from build123d import *

# Parameters (mm, degrees)
F0_W     = 50.8
F0_H     = 38.1
F1_DEPTH = 12.7
F3_DEPTH = 12.7
F5_DEPTH = 12.7
F6_R     = 6.3499999233
F7_DEPTH = 25.401
F8_R     = 6.35
F9_DEPTH = 12.701
F10_R    = 12.7


with BuildPart() as f1:
    # F0 (on Top) → F1 (new body)
    with BuildSketch(Plane.XY):
        Rectangle(F0_W, F0_H)
    extrude(amount=F1_DEPTH)

    # F2 (on face) → F3 (join)
    with BuildSketch(Plane(origin=(0, 19.05, 0), x_dir=(-1, 0, 0), z_dir=(0, 1, 0))):
        with BuildLine():
            ThreePointArc((-12.7, 26.0490588844), (-17.3287683055, 17.7369875968), (-25.4, 12.7))
            Line((-25.4, 12.7), (-12.7, 12.7))
            Line((-12.7, 12.7), (12.7, 12.7))
            Line((12.7, 12.7), (25.4, 12.7))
            ThreePointArc((25.4, 12.7), (17.3287683055, 17.7369875968), (12.7, 26.0490588844))
            Line((12.7, 26.0490588844), (12.7, 69.85))
            ThreePointArc((12.7, 69.85), (0, 57.15), (-12.7, 69.85))
            Line((-12.7, 69.85), (-12.7, 26.0490588844))
        make_face()
        with BuildLine():
            ThreePointArc((12.7, 69.85), (0, 82.55), (-12.7, 69.85))
            ThreePointArc((-12.7, 69.85), (0, 57.15), (12.7, 69.85))
        make_face()
    extrude(amount=-F3_DEPTH)

    # F4 (on face) → F5 (join)
    with BuildSketch(Plane.XZ.offset(-6.35)):
        with BuildLine():
            ThreePointArc((-12.7, 69.85), (0, 57.15), (12.7, 69.85))
            ThreePointArc((12.7, 69.85), (0, 82.55), (-12.7, 69.85))
        make_face()
    extrude(amount=F5_DEPTH)

    # F6 (on face) → F7 (cut, through all)
    with BuildSketch(Plane.XZ.offset(6.35)):
        with Locations((0, 69.85)):
            Circle(F6_R)
    extrude(amount=-F7_DEPTH, mode=Mode.SUBTRACT)

    # F8 (on face) → F9 (cut, through all)
    with BuildSketch(Plane.XY.offset(12.7)):
        with Locations((-12.7, -6.35)):
            Circle(F8_R)
        with Locations((12.7, -6.35)):
            Circle(F8_R)
    extrude(amount=-F9_DEPTH, mode=Mode.SUBTRACT)

    # F10
    f10_edges = [f1.edges().sort_by_distance(p)[0] for p in [
        (-25.4, -19.05, 6.35),
        (25.4, -19.05, 6.35),
    ]]
    fillet(f10_edges, radius=F10_R)


solid = f1.part
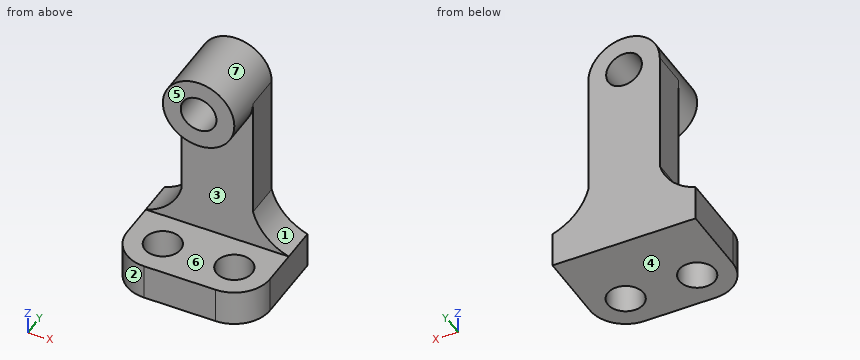
Design review of the part built by this model. Coordinates are the model's own, in mm. Face numbers are marked on the shaded views. A direction names the side the tool comes from. Give positions to 0.01 mm unless a question says otherwise; leave off trailing zeros. Write each loop counter-clockwise with the first axis right and the second up, starting at its lowest first coordinate (ties: lowest second). Pieces come first, ordered by that corner, then holes. Notation, with made-up numbers: M -1.5,-1 L 11.5,-1 A11 cw 11.5,19 Z; hole C 24,62 d8. An arc over 180 degrees is marked long. Return JSON: item names as keys, results as strings. Group by question number.
Item 1: Clearance check with flat-ended pins moving along their axes: pin 1 Ø2 at (y, z) = (4, 32) entering from +X; pin 2 Ø6.5 at (y, z) = (14, 39) entering from +X; pin 3 Ø16.5 at (x, z) = (0, 69.85) entering from -Y; pin 4 Ø14 at (y, z) = (11, 48) entering from -X. State where each tip first meets the part, or that it passes through.
Item 2: The part is to be moulded in two halves that separate along Z. For the marked faces 1, 2, 3 and 4, say which applies: pulls with the +Z half, pulls with the -Z half, needs draft (parallel to the pull), parting line crosses it, or undercut.
Item 3: Take a section at A-A (y = 1.5). Give the boundary of the cut face in (x, z), plus the area to 3 significant figures.
Item 4: Take a section at B-B (x = 0). Give the boundary of the cut face in (y, z), plus the area to 3 significant figures.
Item 5: Take a section at D-D (y = -11.5). Give the boundary of the cut face in (x, z), plus the area to 3 significant figures.
Item 6: Tool access review of the marked faces 5, 6 and 7: name each direction out of +Z, -Z, +X, -X, +Y, -Y from which nothing blocks a thin tool from reaching the whole face with its end or side.
Item 7: Wall thickness on line 1 along X through (y, z) = (-6, 6); line 2 along Z through (x, y) = (0, 12); line 3 along X through (y, z) = (-11, 9): over which ranges is each line inside the solid? List them lowest first.
Item 8: Take a section at C-C (y = 16). Give the boundary of the cut face in (x, z), plus the area to 3 significant figures.
Return value:
{
 "1": {"pin 1": "passes through", "pin 2": "stops at x = 12.7", "pin 3": "stops at y = -6.35", "pin 4": "stops at x = -12.7"},
 "2": {"face 1": "pulls with the +Z half", "face 2": "needs draft", "face 3": "undercut", "face 4": "pulls with the -Z half"},
 "3": {"outline": "M -25.4,0 L 25.4,0 L 25.4,12.7 L -25.4,12.7 Z; C 0,69.85 d25.4; hole C 0,69.85 d12.7", "area": "1,030 mm2"},
 "4": {"outline": "M -19.05,0 L 19.05,0 L 19.05,63.5 L -6.35,63.5 L -6.35,57.15 L 6.35,57.15 L 6.35,12.7 L -19.05,12.7 Z; M -6.35,76.2 L 19.05,76.2 L 19.05,82.55 L -6.35,82.55 Z", "area": "1,370 mm2"},
 "5": {"outline": "M -24.31,0 L -16.41,0 L -16.41,12.7 L -24.31,12.7 Z; M -8.99,0 L 8.99,0 L 8.99,12.7 L -8.99,12.7 Z; M 16.41,0 L 24.31,0 L 24.31,12.7 L 16.41,12.7 Z", "area": "429 mm2"},
 "6": {"face 5": "+Z, +X, -X, -Y", "face 6": "+X, -X, -Y", "face 7": "-Y"},
 "7": {"line 1": "x = -25.4 to -19.04, -6.36 to 6.36, 19.04 to 25.4", "line 2": "z = 0 to 63.5, 76.2 to 82.55", "line 3": "x = -24.52 to -17.02, -8.38 to 8.38, 17.02 to 24.52"},
 "8": {"outline": "M -25.4,0 L 25.4,0 L 25.4,12.7 A19.05 cw 12.7,26.05 L 12.7,69.85 A12.7 ccw -12.7,69.85 L -12.7,26.05 A19.05 cw -25.4,12.7 Z; hole C 0,69.85 d12.7", "area": "2,330 mm2"}
}
